CAD build for the part. Positions are in the model's coordinates, mm. A direction names the side the tool comes from. Round coordinates to 2 decimals unless told otherwise and drop trailing zeros. Order: outer loops, then holes, each group sorted by start corner. A loop starts at its lowest first (then second) coordinate and runs counter-clockwise, first axis right, second up. Notation, with made-up numbers: M 89.25,56 L 100.25,56 A28 cw 100.25,75 Z; hole C 35,10.25 d2. An arc over 180 degrees is marked long. Put each result on its own line as item: value.
Autodesk Fusion 360 part; units mm, degrees
sketch "Sketch1" plane through (0, 0, 0) normal (0, 0, 1) x (1, 0, 0)
  line L0 (-25, 25) -> (25, 25)
  line L1 (25, 25) -> (25, -25)
  line L2 (25, -25) -> (-25, -25)
  line L3 (-25, -25) -> (-25, 25)
  line L4 (-25, 25) -> (25, -25) construction
  line L5 (25, 25) -> (-25, -25) construction
  dimension "d1" = 50
  dimension "d2" = 50
extrude "Extrude1" add sketch "Sketch1" along normal blind 20
sketch "Sketch2" plane through (0, 0, 20) normal (0, 0, 1) x (1, 0, 0)
  line L0 (-25, -25) -> (25, -25)
  line L1 (25, -25) -> (25, 25)
  line L2 (25, 25) -> (-25, 25)
  line L3 (-25, 25) -> (-25, -25)
  line L4 (21.2132, 0) -> (0, -21.2132)
  line L5 (0, -21.2132) -> (-21.2132, 0)
  line L6 (-21.2132, 0) -> (0, 21.2132)
  line L7 (0, 21.2132) -> (21.2132, 0)
  line L8 (0, -25) -> (0, 25) construction
  line L9 (0, -21.2132) -> (0, 21.2132) construction
  line L10 (21.2132, 0) -> (-21.2132, 0) construction
  line L11 (25, 0) -> (-25, 0) construction
  dimension "d5" = 30
  dimension "d6" = 30
extrude "Extrude2" add sketch "Sketch2" along normal blind 1.5 contours L4 L5 L6 L7
sketch "Sketch3" plane through (0, 0, 21.5) normal (0, 0, 1) x (1, 0, 0)
  line L0 (0, 21.2132) -> (-21.2132, 0)
  line L1 (-21.2132, 0) -> (0, -21.2132)
  line L2 (0, -21.2132) -> (21.2132, 0)
  line L3 (21.2132, 0) -> (0, 21.2132)
  circle A0 centre (0, 0) radius 13 construction
  circle A1 centre (0, -13) radius 2.5
  circle A2 centre (-13, 0) radius 2.5
  circle A3 centre (0, 13) radius 2.5
  circle A4 centre (13, 0) radius 2.5
  dimension "d9" = 26
  dimension "d10" = 5
hole "Hole1" at (-13, 0, 21.5) at (0, -13, 21.5) at (0, 13, 21.5) at (13, 0, 21.5) direction (0, 0, -1) diameter 4 depth 3 tip angle 180
sketch "Sketch4" plane through (0, 0, 21.5) normal (0, 0, 1) x (1, 0, 0)
  circle A0 centre (0, 13) radius 2
  circle A1 centre (-13, 0) radius 2
  circle A2 centre (0, -13) radius 2
  circle A3 centre (13, 0) radius 2
  line L0 (0, 21.2132) -> (-21.2132, 0)
  line L1 (-21.2132, 0) -> (0, -21.2132)
  line L2 (0, -21.2132) -> (21.2132, 0)
  line L3 (21.2132, 0) -> (0, 21.2132)
  line L4 (4.5, -7.5) -> (-4.5, -7.5)
  line L5 (-7.5, -4.5) -> (-7.5, 4.5)
  line L6 (-4.5, 7.5) -> (4.5, 7.5)
  line L7 (7.5, 4.5) -> (7.5, -4.5)
  line L8 (7.5, -7.5) -> (-7.5, 7.5) construction
  line L9 (-7.5, -7.5) -> (7.5, 7.5) construction
  arc A4 (4.5, -7.5) -> (7.5, -4.5) centre (4.5, -4.5) ccw
  arc A5 (-7.5, -4.5) -> (-4.5, -7.5) centre (-4.5, -4.5) ccw
  arc A6 (7.5, 4.5) -> (4.5, 7.5) centre (4.5, 4.5) ccw
  arc A7 (-4.5, 7.5) -> (-7.5, 4.5) centre (-4.5, 4.5) ccw
  dimension "d14" = 15
  dimension "d15" = 15
  dimension "d16" = 3
  dimension "d17" = 3
  dimension "d18" = 3
  dimension "d19" = 3
extrude "Extrude3" add sketch "Sketch4" along normal blind 1.5 contours L4 L5 L6 L7 A4 A5 A6 A7
sketch "Sketch5" plane through (0, 0, 23) normal (0, 0, 1) x (1, 0, 0)
  arc A0 (7.5, 4.5) -> (4.5, 7.5) centre (4.5, 4.5) ccw
  line L0 (4.5, 7.5) -> (-4.5, 7.5)
  arc A1 (-4.5, 7.5) -> (-7.5, 4.5) centre (-4.5, 4.5) ccw
  line L1 (-7.5, 4.5) -> (-7.5, -4.5)
  arc A2 (-7.5, -4.5) -> (-4.5, -7.5) centre (-4.5, -4.5) ccw
  line L2 (-4.5, -7.5) -> (4.5, -7.5)
  arc A3 (4.5, -7.5) -> (7.5, -4.5) centre (4.5, -4.5) ccw
  line L3 (7.5, -4.5) -> (7.5, 4.5)
  circle A4 centre (0, 0) radius 6 construction
  line L4 (6.6213, -6.6213) -> (-6.6213, 6.6213) construction
  line L5 (-6.6213, -6.6213) -> (6.6213, 6.6213) construction
  circle A5 centre (0, 0) radius 1.5
  circle A6 centre (-4.2426, -4.2426) radius 1.5
  circle A7 centre (4.2426, -4.2426) radius 1.5
  circle A8 centre (4.2426, 4.2426) radius 1.5
  circle A9 centre (-4.2426, 4.2426) radius 1.5
  dimension "d22" = 12
  dimension "d23" = 3
hole "Hole2" at (-4.2426, -4.2426, 23) at (4.2426, -4.2426, 23) at (-4.2426, 4.2426, 23) at (4.2426, 4.2426, 23) at (0, 0, 23) direction (0, 0, -1) diameter 3 depth 5 tip angle 180
sketch "Sketch6" plane through (0, 0, 20) normal (0, 0, 1) x (1, 0, 0)
  line L0 (0, 21.2132) -> (21.2132, 0)
  line L1 (21.2132, 0) -> (0, -21.2132)
  line L2 (0, -21.2132) -> (-21.2132, 0)
  line L3 (-21.2132, 0) -> (0, 21.2132)
  line L4 (-25, -25) -> (25, -25)
  line L5 (25, -25) -> (25, 25)
  line L6 (25, 25) -> (-25, 25)
  line L7 (-25, 25) -> (-25, -25)
  line L8 (-25, -25) -> (-10.6066, -10.6066) construction
  line L9 (-19.6648, -22.9418) -> (-12.6648, -15.9418)
  arc A0 (-12.6648, -15.9418) -> (-15.9418, -12.6648) centre (-14.3033, -14.3033) ccw
  line L10 (-15.9418, -12.6648) -> (-22.9418, -19.6648)
  arc A1 (-22.9418, -19.6648) -> (-19.6648, -22.9418) centre (-21.3033, -21.3033) ccw
  line L11 (-21.3033, -21.3033) -> (-14.3033, -14.3033) construction
  line L12 (12.6648, -15.9418) -> (19.6648, -22.9418)
  arc A2 (19.6648, -22.9418) -> (22.9418, -19.6648) centre (21.3033, -21.3033) ccw
  line L13 (22.9418, -19.6648) -> (15.9418, -12.6648)
  arc A3 (15.9418, -12.6648) -> (12.6648, -15.9418) centre (14.3033, -14.3033) ccw
  line L14 (15.9418, 12.6648) -> (22.9418, 19.6648)
  arc A4 (22.9418, 19.6648) -> (19.6648, 22.9418) centre (21.3033, 21.3033) ccw
  line L15 (19.6648, 22.9418) -> (12.6648, 15.9418)
  arc A5 (12.6648, 15.9418) -> (15.9418, 12.6648) centre (14.3033, 14.3033) ccw
  line L16 (-12.6648, 15.9418) -> (-19.6648, 22.9418)
  arc A6 (-19.6648, 22.9418) -> (-22.9418, 19.6648) centre (-21.3033, 21.3033) ccw
  line L17 (-22.9418, 19.6648) -> (-15.9418, 12.6648)
  arc A7 (-15.9418, 12.6648) -> (-12.6648, 15.9418) centre (-14.3033, 14.3033) ccw
  dimension "d28" = 360
extrude "Extrude4" cut sketch "Sketch6" against normal blind 3 contours L9 A0 L10 A1 | L12 A2 L13 A3 | L14 A4 L15 A5 | L16 A6 L17 A7
Item 1: Pin check, flat tips, straight feed: P1, Ø3.5, axis at x = 20, y = -17, coming from the +Z side; P2, Ø2.5, axis at x = 0, y = -13, coming from the +Z side; P3, Ø0.9, axis at x = 0, y = 0.5, coming from the +Z side. Stop position of each tip, or through.
Answers below:
P1: z = 20
P2: z = 18.5
P3: z = 18
Item 2: Mould opens along X. For faces 5 (the flat face through (-18, -18, 17)), 6 (the flat face through (10.755, -10.458, 20.74)), 7 (the flat face through (0, -2, 23)) say: pulls with the +X half, pulls with the -X half, needs draft (parallel to the pull), parting line crosses it, or undercut.
Answers below:
face 5: undercut
face 6: pulls with the +X half
face 7: needs draft
Item 3: Tool access for faces 1 (the cylindrical face through (-6.64, 6.6, 22.24)), 2 (the flat face through (0, -25, 10)), 3 (the flat face through (-16.116, 19.393, 18.521)), 4 (the cylindrical face through (-6.6, -6.64, 22.24)): list every direction of +Z, -Z, +X, -X, +Y, -Y with a clear straight run to the whole face (end or side of a thin tool).
Answers below:
face 1: +Z, -X, +Y
face 2: +Z, -Z, +X, -X, -Y
face 3: +Z
face 4: +Z, -X, -Y
Item 4: Probe line 1 along Y through (x, z) = (0, 19.95); line 2 along Y through (x, z) = (13, 17.25); line 3 along Z through (x, y) = (10, -7). List the from-to ranges inside material, lowest first. Write a range as [from, to].
Answers below:
line 1: [-25, -15], [-11, -1.5], [1.5, 11], [15, 25]
line 2: [-25, -16.28], [-12.39, 12.39], [16.28, 25]
line 3: [0, 21.5]
Item 5: Band-saw the part on A-A on y = 18.5. Give the cut face in (x, z).
Answers below:
outline: M -25,0 L 25,0 L 25,20 L 21.78,20 L 21.78,17 L 15.22,17 L 15.22,20 L 2.71,20 L 2.71,21.5 L -2.71,21.5 L -2.71,20 L -15.22,20 L -15.22,17 L -21.78,17 L -21.78,20 L -25,20 Z
